Geometry check sheet. Reference: the model listing, model coordinates, mm. Face numbers are marked on the shaded views. A direction names the side the tool comes from. Round coordinates to 2 decimals unless told otherwise and drop trailing zeros. Loops run counter-clockwise (first coordinate to the right, second up) from the corner with the lowest first, then second, coordinate; pieces in that order, holes last. Notation, with made-up numbers: (85.5, 50.25) - (136.5, 50.25) arc R13 cw to (136.5, 69.25) - close; hole circle Ø8 at (21, 64). An arc over 180 degrees is marked (long way). Answer as CSV lines item,"result". Start each with the question number.
1) Draft check along Z on the marked faces 1, 2 and 3. Enter one of: released by +Z, released by -Z, zero draft, split by the parting line, or undercut.
2) Thickness scan on line 1 along Z through (x, y) = (0, 2.7) (3 decimals); line 2 along X through (y, z) = (4.5, -14.5); line 3 along Y through (x, z) = (5, -8.5). Record the ranges inside material, lowest first.
3) Cross-section at D-D on y = 5. Record the boundary of the cut face in (x, z) (1 decimal), and give its area (3 significant figures).
4) Cross-section at A-A on z = 0. Record the boundary of the cut face in (x, y) (3 decimals).
5) Cross-section at C-C on x = -9.5. Record the boundary of the cut face in (y, z) (3 decimals), and give its area (3 significant figures).
6) Access from +Z, -Z, +X, -X, +Y, -Y to the whole of each face (thin tool, end or side, straight path). Record for the marked faces 4 and 5.
7) Cross-section at B-B on y = 3. Record the boundary of the cut face in (x, z) (3 decimals), and give its area (3 significant figures).
8) Depth check by flat-ended pin: P1, Ø4.5, axis at x = 0, z = 0, coming from the +Y side; P2, Ø14.5, axis at x = 0, z = 0, coming from the +Y side; P3, Ø5.5, axis at x = 1, z = -1.5, coming from the +Y side. Enter the tip coordinate at first touch or a pass-through.
from build123d import *

# Parameters (mm, degrees)
SKETCH1_W                       = 35.56
SKETCH1_H                       = 36.83
BOSS_EXTRUDE1_DEPTH             = 10
SKETCH5_R                       = 1.905
BOSS_EXTRUDE2_DEPTH             = 2
M2X0_4_TAPPED_HOLE1_D           = 1.6
M2X0_4_TAPPED_HOLE1_CSINK_D     = 2.05
M2X0_4_TAPPED_HOLE1_CSINK_ANGLE = 90


with BuildPart() as part:
    # Sketch1 → Boss-Extrude1 (new body)
    with BuildSketch(Plane(origin=(0, 0, 0), x_dir=(1, 0, 0), z_dir=(0, 1, 0))):
        Rectangle(SKETCH1_W, SKETCH1_H)
    extrude(amount=BOSS_EXTRUDE1_DEPTH)

    # Sketch4 → CBORE for 1/4 Socket Head Cap Screw1 (revolve, cut)
    with BuildSketch(Plane(origin=(0, 10, 0), x_dir=(0, 0, 1), z_dir=(1, 0, 0))):
        Polygon((0, 0), (0, 10), (3.57124, 10), (3.57124, 6.35), (5.55625, 6.35), (5.55625, 0.635), (6.19125, 0), align=None)
    revolve(axis=Axis((0, 16.35, 0), (0, -1, 0)), mode=Mode.SUBTRACT)

    # Sketch5 → Boss-Extrude2 (add)
    with BuildSketch(Plane(origin=(0, 10, 0), x_dir=(1, 0, 0), z_dir=(0, 1, 0))):
        with Locations(Location((-14.478, 15.113, 0), (0, 0, 270))):
            Circle(SKETCH5_R)
        with Locations(Location((14.478, 15.113, 0), (0, 0, 270))):
            Circle(SKETCH5_R)
        with Locations(Location((1.778, -15.113, 0), (0, 0, 270))):
            Circle(SKETCH5_R)
    extrude(amount=BOSS_EXTRUDE2_DEPTH)

    # M2x0.4 Tapped Hole1 (through all)
    with Locations(Plane(origin=(0, 12, 0), x_dir=(1, 0, 0), z_dir=(0, 1, 0))):
        with Locations((-14.478, 15.113), (14.478, 15.113), (1.778, -15.113)):
            CounterSinkHole(M2X0_4_TAPPED_HOLE1_D / 2, M2X0_4_TAPPED_HOLE1_CSINK_D / 2, counter_sink_angle=M2X0_4_TAPPED_HOLE1_CSINK_ANGLE)


solid = part.part
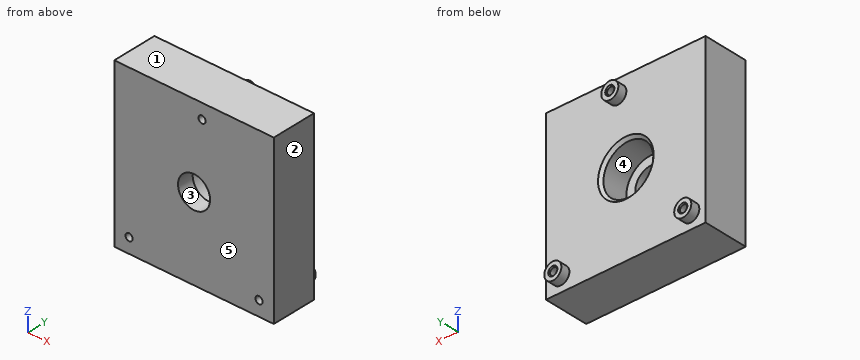
Answer block:
1,face 1,"released by +Z"
1,face 2,"zero draft"
1,face 3,"undercut"
2,line 1,"z = -18.415 to -3.571, 3.571 to 18.415"
2,line 2,"x = -17.78 to -14.99, -13.96 to 13.96, 14.99 to 17.78"
2,line 3,"y = 0 to 10"
3,outline,"(-17.8, -18.4) - (17.8, -18.4) - (17.8, 18.4) - (-17.8, 18.4) - close; hole circle Ø1.6 at (-14.5, -15.1); hole circle Ø11.1 at (0, 0); hole circle Ø1.6 at (1.8, 15.1); hole circle Ø1.6 at (14.5, -15.1)"
3,area,"1,210 mm^2"
4,outline,"(-17.78, 0) - (-3.571, 0) - (-3.571, 3.65) - (-5.556, 3.65) - (-5.556, 9.365) - (-6.191, 10) - (-17.78, 10) - close; (3.571, 0) - (17.78, 0) - (17.78, 10) - (6.191, 10) - (5.556, 9.365) - (5.556, 3.65) - (3.571, 3.65) - close"
5,outline,"(0, -18.415) - (10, -18.415) - (10, 18.415) - (0, 18.415) - close"
5,area,"368 mm^2"
6,face 4,"+Y"
6,face 5,"+Z, -Z, +X, -X, -Y"
7,outline,"(-17.78, -18.415) - (17.78, -18.415) - (17.78, 18.415) - (-17.78, 18.415) - close; hole circle Ø1.6 at (-14.478, -15.113); hole circle Ø7.142 at (0, 0); hole circle Ø1.6 at (1.778, 15.113); hole circle Ø1.6 at (14.478, -15.113)"
7,area,"1,260 mm^2"
8,P1,"passes through"
8,P2,"stops at y = 10"
8,P3,"stops at y = 3.65"
